Part model, mm, in its own coordinate system. A direction names the side the tool comes from. Coordinates: 2 decimals unless noted, no trailing zeros. Order: outer loops, then holes, each group sorted by start corner. A loop starts at its lowest first (then second) coordinate and runs counter-clockwise, first axis right, second up.
from build123d import *

# Parameters (mm, degrees)
F0_W         = 52
F0_H         = 52
F0_R         = 24.7301056407
F1_DEPTH     = 92
F2_W         = 38
F2_H         = 35
F3_DEPTH     = 52.001
F4_R         = 5
F5_T4_ANGLE  = 79.1651275765
F5_T9_ANGLE  = 158.3519759407
F5_T15_ANGLE = 79.1651275765
F6_R         = 1.45
F7_DEPTH     = 10
F8_R         = 1.45
F9_DEPTH     = 52.001
F10_W        = 25
F10_H        = 26
F11_DEPTH    = 92.0010001
F12_W        = 10
F12_H        = 10
F12_R        = 1.75
F13_DEPTH    = 10
F14_R        = 4.99999
F15_R        = 3
F16_DEPTH    = 4


# Not quite as in the source:
# - a fillet or chamfer that OpenCascade refuses, or shapes differently, is made with other operations: its cross-section is extruded or revolved along the edge and cut away or added
# - a fillet or chamfer is up to 0.001 mm smaller than in the source, because OpenCascade refuses the exact size


with BuildPart() as f1:
    # F0 (on Top) → F1 (new body)
    with BuildSketch(Plane.XY):
        Rectangle(F0_W, F0_H)
        Circle(F0_R, mode=Mode.SUBTRACT)
    extrude(amount=F1_DEPTH)

    # F2 (on face) → F3 (cut, through all)
    with BuildSketch(Plane(origin=(-26, 0, 0), x_dir=(0, -1, 0), z_dir=(-1, 0, 0))):
        with Locations((0, 74.5)):
            Rectangle(F2_W, F2_H)
    extrude(amount=-F3_DEPTH, mode=Mode.SUBTRACT)

    # F4
    f4_edges = [f1.edges().sort_by_distance(p)[0] for p in [
        (-26, 26, 46),
        (-26, -26, 46),
        (26, 26, 46),
        (26, -26, 46),
    ]]
    fillet(f4_edges, radius=F4_R)

    # F5: fillet of radius 5 on 3 edges, made by hand


with BuildPart() as f5_tool2:
    # F5_s3 → F5_t4 (revolve)
    with BuildSketch(Plane.XZ):
        with BuildLine():
            ThreePointArc((24.7301056407, 52), (26.1945717348, 55.5355339059), (29.7301056407, 57))
            Line((29.7301056407, 57), (24.7301056407, 57))
            Line((24.7301056407, 57), (24.7301056407, 52))
        make_face()
    revolve(axis=Axis((0, 0, 57), (0, 0, -1)), revolution_arc=F5_T4_ANGLE)

    split(bisect_by=Plane.XZ.offset(19), keep=Keep.BOTTOM)


with BuildPart() as f1_1:
    add(f1.part)

    # F5_t1: cut F5_tool2
    add(f5_tool2.part, mode=Mode.SUBTRACT)


with BuildPart() as f5_tool7:
    # F5_s8 → F5_t9 (revolve)
    with BuildSketch(Plane(origin=(0, 0, 0), x_dir=(0, 0, 1), z_dir=(0.982208635, -0.1877929639, 0))):
        with BuildLine():
            ThreePointArc((52, 24.7301056407), (55.5355339059, 26.1945717348), (57, 29.7301056407))
            Line((57, 29.7301056407), (57, 24.7301056407))
            Line((57, 24.7301056407), (52, 24.7301056407))
        make_face()
    revolve(axis=Axis((0, 0, 57), (0, 0, -1)), revolution_arc=F5_T9_ANGLE)

    split(bisect_by=Plane.XZ.offset(-19), keep=Keep.TOP)

    split(bisect_by=Plane.XZ.offset(19), keep=Keep.BOTTOM)


with BuildPart() as f1_2:
    add(f1_1.part)

    # F5_t6: cut F5_tool7
    add(f5_tool7.part, mode=Mode.SUBTRACT)


with BuildPart() as f5_tool13:
    # F5_s14 → F5_t15 (revolve)
    with BuildSketch(Plane(origin=(0, 0, 0), x_dir=(0, 0, 1), z_dir=(-0.9821730213, 0.1879791378, 0))):
        with BuildLine():
            ThreePointArc((52, 24.7301056407), (55.5355339059, 26.1945717348), (57, 29.7301056407))
            Line((57, 29.7301056407), (57, 24.7301056407))
            Line((57, 24.7301056407), (52, 24.7301056407))
        make_face()
    revolve(axis=Axis((0, 0, 57), (0, 0, -1)), revolution_arc=F5_T15_ANGLE)

    split(bisect_by=Plane.XZ.offset(-19), keep=Keep.TOP)


with BuildPart() as f1_3:
    add(f1_2.part)

    # F5_t12: cut F5_tool13
    add(f5_tool13.part, mode=Mode.SUBTRACT)

    # F6 (on face) → F7 (cut)
    with BuildSketch(Plane.XY):
        with Locations((-20, -20)):
            Circle(F6_R)
        with Locations((20, -20)):
            Circle(F6_R)
        with Locations((20, 20)):
            Circle(F6_R)
        with Locations((-20, 20)):
            Circle(F6_R)
    extrude(amount=F7_DEPTH, mode=Mode.SUBTRACT)

    # F8 (on face) → F9 (cut, through all)
    with BuildSketch(Plane(origin=(0, 26, 0), x_dir=(-1, 0, 0), z_dir=(0, 1, 0))):
        with Locations((-10, 63)):
            Circle(F8_R)
        with Locations((10, 63)):
            Circle(F8_R)
    extrude(amount=-F9_DEPTH, mode=Mode.SUBTRACT)

    # F10 (on face) → F11 (cut, through all)
    with BuildSketch(Plane.XY):
        with Locations((-28.625, 0)):
            Rectangle(F10_W, F10_H)
    extrude(amount=F11_DEPTH, mode=Mode.SUBTRACT)

    # F12 (on face) → F13 (join)
    with BuildSketch(Plane.XY.offset(92)):
        with Locations((0, -31)):
            Rectangle(F12_W, F12_H)
        with Locations((0, -31)):
            Circle(F12_R, mode=Mode.SUBTRACT)
        with Locations((0, 31)):
            Rectangle(F12_W, F12_H)
        with Locations((0, 31)):
            Circle(F12_R, mode=Mode.SUBTRACT)
    extrude(amount=-F13_DEPTH)

    # F14 (radius 5 in the source; OpenCascade refuses exactly that, so slightly less here)
    f14_edges = [f1_3.edges().sort_by_distance(p)[0] for p in [
        (-5, -26, 87),
        (5, -26, 87),
        (-5, 26, 87),
        (5, 26, 87),
        (5, 36, 87),
        (-5, 36, 87),
        (-5, -36, 87),
        (5, -36, 87),
    ]]
    fillet(f14_edges, radius=F14_R)

    # F15 (on face) → F16 (cut)
    with BuildSketch(Plane(origin=(0, 0, 82), x_dir=(1, 0, 0), z_dir=(0, 0, -1))):
        with Locations((0, 31.0749467462)):
            Circle(F15_R)
        with Locations((0, -31)):
            Circle(F15_R)
    extrude(amount=-F16_DEPTH, mode=Mode.SUBTRACT)


solid = f1_3.part
Q1. Cut at C-C on z = 17. Write the cut outline in (x, y).
Results list:
outline: (-26, -21) arc R5 ccw to (-21, -26) - (21, -26) arc R5 ccw to (26, -21) - (26, 21) arc R5 ccw to (21, 26) - (-21, 26) arc R5 ccw to (-26, 21) - (-26, 13) - (-21.04, 13) arc R24.73 cw (long way) to (-21.04, -13) - (-26, -13) - close
Q2. Pin check, flat tips, straight feed: pin 1 Ø12 at (y, z) = (21.5, 22.5) entering from +X; pin 2 Ø5 at (x, z) = (19.5, 63) entering from -Y; pin 3 Ø2.5 at (x, y) = (24.5, 17.5) entering from +Z; pin 4 Ø8 at (x, z) = (19, 70) entering from +Y. Stop position of each tip, or through.
Results list:
pin 1: stops at x = 26
pin 2: stops at y = -26
pin 3: stops at z = 57
pin 4: stops at y = 26
Q3. Wall check: line 1 along Y through (x, z) = (0, 84.05); line 2 along Y through (x, z) = (0, 89.4); line 3 along Z through (x, y) = (10, 24). Give the ranges that are in metal, low to high.
Results list:
line 1: y = -36 to -34.07, -28.07 to -24.73, 24.73 to 28, 34 to 36
line 2: y = -36 to -32.75, -29.25 to -24.73, 24.73 to 29.25, 32.75 to 36
line 3: z = 0 to 61.55, 64.45 to 92
Q4. Mould opens along Z. For faces 1 (the face through (4, -34, 87)), 2 (the face through (-11.339, -24.385, 62.445)), 3 (the face through (0, -26, 92)) say: pulls with the +Z half, pulls with the -Z half, needs draft (parallel to the pull), parting line crosses it, or undercut.
Results list:
face 1: needs draft
face 2: undercut
face 3: pulls with the +Z half
Q5. Which spindle directions (+Z, -Z, +X, -X, +Y, -Y) get a long thin tool onto all of the face, cutting with end or side? Do faces 4 (the face through (-25, 18, 57)), 5 (the face through (-0.65, 33.93, 83.97)), 6 (the face through (-25, -24, 47)), 7 (the face through (-0.1, -27.6, 82)). Say none if no direction does.
Results list:
face 4: +Z, +X, -X
face 5: -Z
face 6: +Z, -Z, -X, -Y
face 7: -Z, +X, -X, -Y
Q6. Cut at A-A on z = 6. Write the cut outline in (x, y).
Results list:
outline: (-26, -21) arc R5 ccw to (-21, -26) - (21, -26) arc R5 ccw to (26, -21) - (26, 21) arc R5 ccw to (21, 26) - (-21, 26) arc R5 ccw to (-26, 21) - (-26, 13) - (-21.04, 13) arc R24.73 cw (long way) to (-21.04, -13) - (-26, -13) - close; hole circle Ø2.9 at (-20, -20); hole circle Ø2.9 at (-20, 20); hole circle Ø2.9 at (20, -20); hole circle Ø2.9 at (20, 20)
Q7. Cut at B-B on z = 63. Count the separate pieces of the cut face and the enclosed holes in it, and give its area (3 significant figures).
Results list:
separate pieces: 6
enclosed holes: 0
area: 419 mm2
